from build123d import *
from OCP.BRepFilletAPI import BRepFilletAPI_MakeChamfer

# Parameters (mm, degrees)
SKETCH1_W           = 182
SKETCH1_H           = 81.5
BOSS_EXTRUDE1_DEPTH = 22
BOSS_EXTRUDE1_DRAFT = -32
SHELL1_T            = -5
SKETCH2_R           = 1.6
CUT_EXTRUDE1_DEPTH  = 22
CHAMFER1_SIZE       = 4
CHAMFER1_SIZE2      = 5.891470361
SKETCH3_W           = 15
SKETCH3_H           = 5.895892017
BOSS_EXTRUDE2_DEPTH = 8
SKETCH6_W           = 15
SKETCH6_H           = 4
BOSS_EXTRUDE3_DEPTH = 98
SKETCH7_W           = 15
SKETCH7_H           = 4
BOSS_EXTRUDE4_DEPTH = 98
CHAMFER2_SIZE       = 4


with BuildPart() as part:
    # Sketch1 → Boss-Extrude1 (with draft: the straight prism first)
    with BuildSketch(Plane(origin=(0, 0, 0), x_dir=(1, 0, 0), z_dir=(0, 1, 0))):
        Rectangle(SKETCH1_W, SKETCH1_H)
    extrude(amount=BOSS_EXTRUDE1_DEPTH)
    # Boss-Extrude1: the draft: its side faces are tilted about the plane it starts from
    boss_extrude1_sides = [part.faces().sort_by_distance(p)[0] for p in [
        (0, 11, 40.75),
        (91, 11, 0),
        (0, 11, -40.75),
        (-91, 11, 0),
    ]]
    draft(boss_extrude1_sides, Plane(origin=(0, 0, 0), x_dir=(1, 0, 0), z_dir=(0, 1, 0)), BOSS_EXTRUDE1_DRAFT)

    # Shell1
    shell1_openings = [part.faces().sort_by_distance(p)[0] for p in [
        (0, 22, 0),
    ]]
    offset(amount=SHELL1_T, openings=shell1_openings, kind=Kind.INTERSECTION)

    # Sketch2 → Cut-Extrude1 (cut)
    with BuildSketch(Plane(origin=(0, 5, 0), x_dir=(1, 0, 0), z_dir=(0, 1, 0))):
        with Locations(Location((-66.523454743, 24.138454743, 0), (0, 0, 270))):
            Circle(SKETCH2_R)
        with Locations(Location((-66.523454743, -24.141545257, 0), (0, 0, 270))):
            Circle(SKETCH2_R)
        with Locations(Location((8.406545257, 24.138454743, 0), (0, 0, 270))):
            Circle(SKETCH2_R)
        with Locations(Location((16.026545257, -24.141545257, 0), (0, 0, 270))):
            Circle(SKETCH2_R)
        with Locations(Location((46.506545257, 14.618454743, 0), (0, 0, 270))):
            Circle(SKETCH2_R)
    extrude(amount=-CUT_EXTRUDE1_DEPTH, mode=Mode.SUBTRACT)

    # Chamfer1: one chamfer whose edges measure the first distance from different faces: ONE call of the kernel's chamfer builder (chamfer() names one face for all edges)
    chamfer1_edges_1 = [part.edges().sort_by_distance(p)[0] for p in [
        (97.873562871, 11, 47.623562871),
    ]]
    chamfer1_side_1 = [part.faces().sort_by_distance(p)[0] for p in [
        (0, 11.257506349, 47.784470697),
    ]]
    chamfer1_edges_2 = [part.edges().sort_by_distance(p)[0] for p in [
        (-97.873562871, 11, 47.623562871),
    ]]
    chamfer1_side_2 = [part.faces().sort_by_distance(p)[0] for p in [
        (-98.204252581, 11.529214161, 0),
    ]]
    chamfer1_edges_3 = [part.edges().sort_by_distance(p)[0] for p in [
        (-97.873562871, 11, -47.623562871),
    ]]
    chamfer1_side_3 = [part.faces().sort_by_distance(p)[0] for p in [
        (0, 11.257506349, -47.784470697),
    ]]
    chamfer1_edges_4 = [part.edges().sort_by_distance(p)[0] for p in [
        (97.873562871, 11, -47.623562871),
    ]]
    chamfer1_side_4 = [part.faces().sort_by_distance(p)[0] for p in [
        (98.204252581, 11.529214161, 0),
    ]]
    chamfer1 = BRepFilletAPI_MakeChamfer(part.part.solid().wrapped)
    for e in chamfer1_edges_1:
        chamfer1.Add(CHAMFER1_SIZE, CHAMFER1_SIZE2, e.wrapped, chamfer1_side_1[0].wrapped)  # the first distance lies on this face
    for e in chamfer1_edges_2:
        chamfer1.Add(CHAMFER1_SIZE, CHAMFER1_SIZE2, e.wrapped, chamfer1_side_2[0].wrapped)  # the first distance lies on this face
    for e in chamfer1_edges_3:
        chamfer1.Add(CHAMFER1_SIZE, CHAMFER1_SIZE2, e.wrapped, chamfer1_side_3[0].wrapped)  # the first distance lies on this face
    for e in chamfer1_edges_4:
        chamfer1.Add(CHAMFER1_SIZE, CHAMFER1_SIZE2, e.wrapped, chamfer1_side_4[0].wrapped)  # the first distance lies on this face
    add(Compound.cast(chamfer1.Shape()), mode=Mode.REPLACE)

    # Sketch3 → Boss-Extrude2 (add)
    with BuildSketch(Plane(origin=(0, 22, 0), x_dir=(1, 0, 0), z_dir=(0, 1, 0))):
        with Locations((-76.070202855, 51.549179733)):
            Rectangle(SKETCH3_W, SKETCH3_H)
        with Locations((73.929797145, 51.549179733)):
            Rectangle(SKETCH3_W, SKETCH3_H)
        with Locations((-76.070202855, -51.549179733)):
            Rectangle(SKETCH3_W, SKETCH3_H)
        with Locations((73.929797145, -51.549179733)):
            Rectangle(SKETCH3_W, SKETCH3_H)
    extrude(amount=BOSS_EXTRUDE2_DEPTH)

    # Sketch6 → Boss-Extrude3 (add)
    with BuildSketch(Plane(origin=(0, 0, 48.601233725), x_dir=(-1, 0, 0), z_dir=(0, 0, -1))):
        with Locations((-73.929797145, 28)):
            Rectangle(SKETCH6_W, SKETCH6_H)
    extrude(amount=BOSS_EXTRUDE3_DEPTH)

    # Sketch7 → Boss-Extrude4 (add)
    with BuildSketch(Plane(origin=(0, 0, 48.601233725), x_dir=(-1, 0, 0), z_dir=(0, 0, -1))):
        with Locations((76.070202855, 28)):
            Rectangle(SKETCH7_W, SKETCH7_H)
    extrude(amount=BOSS_EXTRUDE4_DEPTH)

    # Chamfer2
    chamfer2_edges = [part.edges().sort_by_distance(p)[0] for p in [
        (-76.070202855, 26, 48.601233725),
        (-76.070202855, 26, -48.601233725),
        (73.929797145, 26, 48.601233725),
        (73.929797145, 26, -48.601233725),
    ]]
    chamfer(chamfer2_edges, length=CHAMFER2_SIZE - 0.0001)  # a hair under: the kernel refuses the full size


solid = part.part
Input: part model. Units: mm. Frame: model coordinates. A direction names the side the tool comes from. Coordinates: 2 decimals unless noted, no trailing zeros. Loops run counter-clockwise (first coordinate to the right, second up) from the corner with the lowest first, then second, coordinate; pieces in that order, holes last. Notation, with made-up numbers: (17.25, 7) - (50.25, 7) arc R18 cw to (50.25, 20) - close; hole circle Ø4 at (-5, 38.25). An arc over 180 degrees is marked (long way). Answer in a Markdown table with one row per item. Add a question column.
Item 1: Access query for faces 5 (the flat face through (-1, 5, -1)), 6 (the flat face through (99.1, 22, -8.3)), 7 (the flat face through (-2, 22, -52)). Directions: +Z, -Z, +X, -X, +Y, -Y. A direction counts if a zero-diameter tool reaches every point of the face in a straight line with its end or side. Return the directions, or none.
Item 2: Mould query, pull axis X, two halves, no side actions, for faces 1 (the flat face through (-68.57, 28, 1)), 2 (the flat face through (-1.384, 13.381, -43.215)), 3 (the flat face through (95.55, 10.85, 44.15)), 4 (the flat face through (-99.01, 22, -12.87)). Classes: released by +X, released by -X, zero draft, split by the parting line, or undercut.
Item 3: Section query A-A on y = 28. Return the cut outline in (x, z).
Item 4: Section query D-D on y = 10. Return the cut outline in (x, z).
Item 5: Section query C-C on z = 19. Return the cut outline in (x, y).
Item 6: Line query: line 1 along Y through (x, z) = (-61, -10); line 2 along X through (y, z) = (20, -10); line 3 along X through (y, z) = (11.5, -9). Output: solid intervals per line, ascending. Write a range as [from, to].
Item 7: Contact query for flat-ended pins moving along their axis: P1, Ø6.5, axis at x = 31, z = -50.5, coming from the +Y side; P2, Ø10, axis at x = 16, y = 25, coming from the +Z side; P3, Ø1.9, axis at x = 46.51, z = -14.62, coming from the +Y side; P4, Ø12, axis at x = -30, y = 9.5, coming from the +Z side. Output: stop coordinate, or through.
Recorded:
| question | item | result |
|---|---|---|
| 1 | face 5 | none |
| 1 | face 6 | +Z, -Z, +X, +Y |
| 1 | face 7 | +Z, -Z, +Y |
| 2 | face 1 | undercut |
| 2 | face 2 | undercut |
| 2 | face 3 | released by +X |
| 2 | face 4 | zero draft |
| 3 | outline | (-83.57, -54.5) - (-68.57, -54.5) - (-68.57, 54.5) - (-83.57, 54.5) - close; (66.43, -54.5) - (81.43, -54.5) - (81.43, 54.5) - (66.43, 54.5) - close |
| 4 | outline | (-97.25, -40.33) - (-92.72, -47) - (90.58, -47) - (97.25, -42.47) - (97.25, 40.33) - (92.72, 47) - (-90.58, 47) - (-97.25, 42.47) - close; hole (-91.35, -41.1) - (91.35, -41.1) - (91.35, 41.1) - (-91.35, 41.1) - close |
| 5 | outline | (-104.75, 22) - (-91, 0) - (91, 0) - (104.75, 22) - (98.85, 22) - (88.23, 5) - (-88.23, 5) - (-98.85, 22) - close; (-83.57, 26) - (-68.57, 26) - (-68.57, 30) - (-83.57, 30) - close; (66.43, 26) - (81.43, 26) - (81.43, 30) - (66.43, 30) - close |
| 6 | line 1 | [0, 5] |
| 6 | line 2 | [-103.5, -97.6], [97.6, 103.5] |
| 6 | line 3 | [-98.19, -92.29], [92.29, 98.19] |
| 7 | P1 | y = 22 |
| 7 | P2 | z = 54.5 |
| 7 | P3 | through |
| 7 | P4 | z = 50.44 |
